Autodesk Inventor part; units mm, degrees
ref_plane "YZ Plane" through (0, 0, 0) normal (1, 0, 0) x (0, 1, 0)
ref_plane "XZ Plane" through (0, 0, 0) normal (0, 1, 0) x (-1, 0, 0)
ref_plane "XY Plane" through (0, 0, 0) normal (0, 0, 1) x (1, 0, 0)
sketch "Sketch1" plane through (0, 0, 0) normal (0, 1, 0) x (-1, 0, 0)
  line L0 (101.6, -101.6) -> (-101.6, -101.6)
  line L1 (-101.6, -101.6) -> (-101.6, 101.6)
  line L2 (-101.6, 101.6) -> (101.6, 101.6)
  line L3 (101.6, 101.6) -> (101.6, -101.6)
  line L4 (96.6, -96.6) -> (-96.6, -96.6)
  line L5 (-96.6, -96.6) -> (-96.6, 96.6)
  line L6 (-96.6, 96.6) -> (96.6, 96.6)
  line L7 (96.6, 96.6) -> (96.6, -96.6)
  line L8 (101.6, 101.6) -> (-40.4, 101.6)
  circle A0 centre (0, 0) radius 86.4
  circle A1 centre (0, 0) radius 109.3376
  line L9 (-40.4, 101.6) -> (-101.6, 40.4)
  line L10 (-45.4, 101.6) -> (-101.6, 45.4)
  line L11 (96.6, 96.6) -> (96.6, 101.6)
  line L12 (-45.4, 101.6) -> (-35.4, 101.6)
  line L13 (-35.4, 101.6) -> (-35.4, 96.6)
  line L14 (-35.4, 96.6) -> (-45.4, 96.6)
  line L15 (-45.4, 96.6) -> (-45.4, 101.6)
  circle A2 centre (0, 0) radius 111.3376
  point P0 (96.6, 51.2168)
  point P1 (101.6, 40.4)
  point P2 (101.6, -40.4)
  point P3 (96.6, -51.2168)
  point P4 (-96.6, 45.4)
  point P5 (-45.4, 96.6)
  dimension "d0" = 203.2
  dimension "d1" = 203.2
  dimension "d2" = 101.6
  dimension "d3" = 101.6
  dimension "d4" = 5
  dimension "d5" = 5
  dimension "d6" = 5
  dimension "d7" = 5
  dimension "d10" = 142
  dimension "d12" = 61.2
  dimension "d14" = 172.8
  dimension "d15" = 5
  dimension "d16" = 5
  dimension "d17" = 10
  dimension "d34" = 2
extrude "Extrusion1" add sketch "Sketch1" along normal blind 3 contours A2 L7 L4 | L4 A1 L7 A2 | L4 A1 L5 L9 L6 L7 | A2 L5 A1 L4 | L4 L5 A2 | A1 L6 A2 L7 | A2 L6 L7
sketch "Sketch5" plane through (0, 3, 0) normal (0, 1, 0) x (1, 0, 0)
  line L0 (-96.6, -96.6) -> (45.4, -96.6)
  circle A0 centre (0, 0) radius 86.4
  line L1 (96.6, -45.4) -> (96.6, 96.6)
  line L2 (96.6, 0) -> (89.1, 0)
  line L3 (89.1, 0) -> (89.1, 10)
  line L4 (89.1, 10) -> (96.6, 10)
  line L5 (96.6, 10) -> (96.6, 0)
  line L6 (89.1, 0) -> (96.6, 0)
  line L7 (96.6, 0) -> (96.6, -10)
  line L8 (96.6, -10) -> (89.1, -10)
  line L9 (89.1, -10) -> (89.1, 0)
  line L10 (0, 0) -> (96.6, 0)
  point P0 (10, -96.6)
  dimension "d52" = 7.5
  dimension "d53" = 7.5
  dimension "d54" = 10
  dimension "d55" = 10
extrude "Extrusion4" add sketch "Sketch5" along normal blind 15 contours L3 L4 L1 L2 | L2 L1 L8 L9
sketch "Sketch7" plane through (89.1, 3, 10) normal (0, 0, 1) x (1, 0, 0)
  line L0 (2, 10) -> (5.5, 10)
  line L1 (5.5, 10) -> (5.5, 3)
  line L2 (5.5, 3) -> (2, 3)
  line L3 (2, 3) -> (2, 10)
  line L4 (7.5, 0) -> (7.5, 15)
  line L5 (0, 0) -> (0, 15)
  line L6 (0, 15) -> (7.5, 15)
  point P0 (-89.1, -3)
  dimension "d56" = 3.5
  dimension "d57" = 2
  dimension "d58" = 2
  dimension "d59" = 5
  dimension "d60" = 7
extrude "Extrusion6" cut sketch "Sketch7" against normal through all
fillet "Fillet7" radius 3.175 2 edges at (96.6, 18, 0) (89.1, 18, 0)
sketch "Sketch8" plane through (0, 3, 0) normal (0, 1, 0) x (1, 0, 0)
  arc A0 (-101.6, -98.425) -> (-98.425, -101.6) centre (-98.425, -98.425) ccw
  line L0 (44.0849, 101.6) -> (-98.425, 101.6)
  line L1 (-101.6, 98.425) -> (-101.6, -98.425)
  line L2 (-101.6, -46.1) -> (-101.6, -76.6)
  line L3 (-96.6, -96.6) -> (-96.6, 96.6)
  line L4 (-96.6, -46.1) -> (-96.6, -76.6)
  line L5 (-101.6, -76.6) -> (-96.6, -76.6)
  line L6 (-101.6, -46.1) -> (-96.6, -46.1)
  line L7 (-98.425, -101.6) -> (101.6, -101.6)
  line L8 (0, 0) -> (-101.6, 0)
  line L9 (-101.6, 46.1) -> (-101.6, 76.6)
  line L10 (-96.6, 46.1) -> (-96.6, 76.6)
  line L11 (-101.6, 76.6) -> (-96.6, 76.6)
  line L12 (-101.6, 46.1) -> (-96.6, 46.1)
  line L13 (-96.6, -76.6) -> (-90.1, -76.6)
  line L14 (-90.1, -76.6) -> (-90.1, -46.1)
  line L15 (-90.1, -46.1) -> (-96.6, -46.1)
  line L16 (-96.6, -46.1) -> (-96.6, -76.6)
  arc A1 (-98.425, 101.6) -> (-101.6, 98.425) centre (-98.425, 98.425) ccw
  line L17 (-101.6, 46.1) -> (-101.6, 76.6)
  line L18 (-96.6, 46.1) -> (-96.6, 76.6)
  line L19 (-101.6, 76.6) -> (-96.6, 76.6)
  line L20 (-101.6, 46.1) -> (-96.6, 46.1)
  line L21 (-96.6, 76.6) -> (-90.1, 76.6)
  line L22 (-90.1, 76.6) -> (-90.1, 46.1)
  line L23 (-90.1, 46.1) -> (-96.6, 46.1)
  line L24 (-96.6, 46.1) -> (-96.6, 76.6)
  line L25 (-96.6, -76.6) -> (-101.6, -76.6)
  line L26 (-101.6, -76.6) -> (-101.6, -74.1)
  line L27 (-101.6, -74.1) -> (-96.6, -74.1)
  line L28 (-96.6, -74.1) -> (-96.6, -76.6)
  line L29 (-96.6, -46.1) -> (-101.6, -46.1)
  line L30 (-101.6, -46.1) -> (-101.6, -48.6)
  line L31 (-101.6, -48.6) -> (-96.6, -48.6)
  line L32 (-96.6, -48.6) -> (-96.6, -46.1)
  line L33 (-96.6, -76.6) -> (-90.1, -76.6)
  line L34 (-90.1, -76.6) -> (-90.1, -74.1)
  line L35 (-90.1, -74.1) -> (-96.6, -74.1)
  line L36 (-96.6, -74.1) -> (-96.6, -76.6)
  line L37 (-96.6, -48.6) -> (-90.1, -48.6)
  line L38 (-90.1, -48.6) -> (-90.1, -46.1)
  line L39 (-90.1, -46.1) -> (-96.6, -46.1)
  line L40 (-96.6, -46.1) -> (-96.6, -48.6)
  line L41 (-96.6, 96.6) -> (-96.6, -96.6)
  line L42 (-90.1, 46.1) -> (-96.6, 46.1)
  line L43 (-96.6, 46.1) -> (-96.6, 48.6)
  line L44 (-96.6, 48.6) -> (-90.1, 48.6)
  line L45 (-90.1, 48.6) -> (-90.1, 46.1)
  line L46 (-90.1, 76.6) -> (-96.6, 76.6)
  line L47 (-96.6, 76.6) -> (-96.6, 74.1)
  line L48 (-96.6, 74.1) -> (-90.1, 74.1)
  line L49 (-90.1, 74.1) -> (-90.1, 76.6)
  point P0 (-98.425, 98.425)
  point P1 (46.1, 101.6)
  point P2 (46.1, 96.6)
  point P3 (76.6, 96.6)
  point P4 (76.6, 101.6)
  point P5 (-46.1, 96.6)
  dimension "d64" = 30.5
  dimension "d65" = 25
  dimension "d66" = 6.5
  dimension "d118" = 2.5
  dimension "d119" = 2.5
  dimension "d120" = 2.5
  dimension "d121" = 2.5
extrude "Extrusion7" cut sketch "Sketch8" against normal through all contours L48 L22 L44 L3 | L37 L14 L35 L3
sketch "Sketch11" plane through (0, 3, 0) normal (0, 1, 0) x (1, 0, 0)
  line L0 (-94, 94) -> (94, 94)
  line L1 (94, 94) -> (94, -94)
  line L2 (94, -94) -> (-94, -94)
  line L3 (-94, -94) -> (-94, 94)
  circle A0 centre (-94, 94) radius 1.5
  circle A1 centre (94, 94) radius 1.5
  circle A2 centre (-94, -94) radius 1.5
  circle A3 centre (94, -39.0849) radius 1.5
  point P0 (0, 0)
  point P1 (0, 0)
  dimension "d98" = 94
  dimension "d99" = 94
  dimension "d100" = 94
  dimension "d101" = 94
  dimension "d102" = 3
  dimension "d103" = 3
  dimension "d104" = 3
  dimension "d105" = 3
extrude "Extrusion8" cut sketch "Sketch11" against normal blind 10 contours L3 A0 L0 | L0 A0 L3 | A1 L1 L0 | L0 L1 A1 | A2 L2 L3 | L3 L2 A2 | A3 L1 | L1 A3
sketch "Sketch12" plane through (0, 3, 0) normal (0, 1, 0) x (1, 0, 0)
  line L0 (-94, 94) -> (94, 94)
  line L1 (94, 94) -> (94, -94)
  line L2 (94, -94) -> (-94, -94)
  line L3 (-94, -94) -> (-94, 94)
  circle A0 centre (-94, 94) radius 2.6
  circle A1 centre (94, 94) radius 2.6
  circle A2 centre (-94, -94) radius 2.6
  circle A3 centre (94, -39.0849) radius 2.6
  point P0 (0, 0)
  point P1 (0, 0)
  point P2 (0, 0)
  dimension "d108" = 94
  dimension "d109" = 94
  dimension "d110" = 94
  dimension "d111" = 94
  dimension "d112" = 5.2
  dimension "d113" = 5.2
  dimension "d114" = 5.2
  dimension "d115" = 5.2
extrude "Extrusion9" cut sketch "Sketch12" against normal blind 1.5 contours L3 A0 L0 | L0 A0 L3 | A1 L1 L0 | L0 L1 A1 | A2 L2 L3 | L3 L2 A2 | A3 L1 | L1 A3
sketch "Sketch13" plane through (0, 3, 0) normal (0, 1, 0) x (1, 0, 0)
  line L0 (94, 96.6) -> (-94, 96.6)
  line L1 (0, 96.6) -> (0, -96.6)
  line L2 (-96.6, -96.6) -> (45.4, -96.6)
  point P0 (0, 0)
ref_plane "Work Plane1" through (0, 3, -96.6) normal (-1, 0, 0) x (0, 0, 1)
sketch "Sketch14" plane through (0, 3, -96.6) normal (-1, 0, 0) x (0, 0, 1)
  line L0 (208.9015, 36.251) -> (-17.5186, 36.251)
  line L1 (-17.5186, 36.251) -> (-17.5186, -18.9911)
  line L2 (-17.5186, -18.9911) -> (208.9015, -18.9911)
  line L3 (208.9015, -18.9911) -> (208.9015, 36.251)
  point P0 (96.6, -3)
extrude "Extrusion10" cut sketch "Sketch14" against normal through all
sketch "Sketch15" plane through (-96.6, 0, -48.6) normal (-1, 0, 0) x (0, 0, 1)
  line L0 (-43.9, 0) -> (-46.9, 0)
  line L1 (141.1, 1.5) -> (141.1, 0)
  line L2 (-43.9, 0) -> (141.1, 0)
  line L3 (141.1, 0) -> (141.1, 1)
  line L4 (141.1, 1) -> (-43.9, 1)
  line L5 (-43.9, 1) -> (-43.9, 0)
  point P0 (48.6, 0)
  dimension "d125" = 1
extrude "Extrusion11" cut sketch "Sketch15" against normal blind 1
equation "\"d1\" = d0"
properties part number "Box_Walls_2"
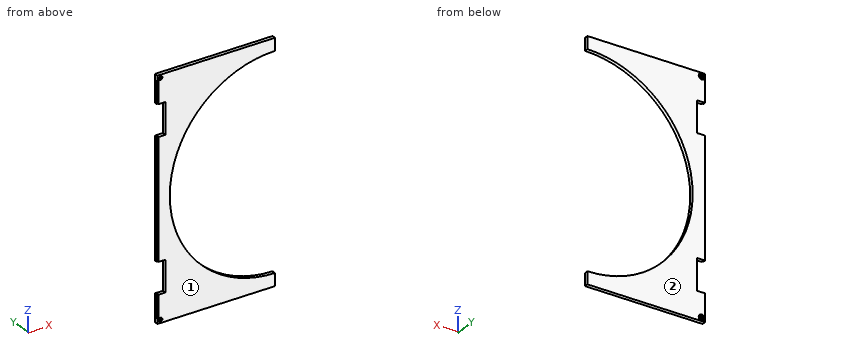
Read the model definition and answer for the solid it produces. Units are mm, in the model's axes. Face numbers are marked on the shaded views. Give positions to 0.01 mm unless a question says otherwise; leave off trailing zeros. Loops run counter-clockwise (first coordinate to the right, second up) from the corner with the lowest first, then second, coordinate; pieces in that order, holes last. Notation, with made-up numbers: (-36.5, -24) - (4.5, -24) arc R28 cw to (4.5, 2) - close; hole circle Ø5 at (46, 25). An arc over 180 degrees is marked (long way). Answer as CSV lines item,"result". Start each with the question number.
1) Find section B-B (x = -57). Write down the section's boundary in (y, z), then the cut area to 3 significant figures.
2) Find section D-D (z = 19.5). Write down the section's boundary in (x, y), then the cut area to 3 significant figures.
3) Straight lines are drawn through the part: L1, parallel to Z at x = -94, y = 1.25; L2, parallel to X at y = 1.05, z = 94; L3, parallel to Z at x = -67, y = 2.3. For each, find the intervals that lie inside material, in ascending order. Write a range as from..to.
4) Each of these flat-tipped pins is pushed along its axis until it touches: pin 1 Ø1.1 at (x, z) = (-96, -86) entering from -Y; pin 2 Ø0.5 at (x, z) = (-96, 79) entering from -Y; pin 3 Ø1.5 at (y, z) = (1.5, 55) entering from -X; pin 4 Ø1.5 at (y, z) = (0.5, -63) entering from +X. Where does it stop, or does it pass through?
5) Determine the mould class of the marked faces 1 and 2 for opening direction Y: released by +Y, released by -Y, zero draft, split by the parting line, or undercut.
6) Find section C-C (z = 0). Write down the section's boundary in (x, y), then the cut area to 3 significant figures.
Findings below:
1,outline,"(0, -96.6) - (3, -96.6) - (3, -64.93) - (0, -64.93) - close; (0, 64.93) - (3, 64.93) - (3, 96.6) - (0, 96.6) - close"
1,area,"190 mm^2"
2,outline,"(-96.6, 1) - (-95.6, 1) - (-95.6, 0) - (-84.17, 0) - (-84.17, 3) - (-96.6, 3) - close"
2,area,"36.3 mm^2"
3,L1,"-96.6..-95.5, -92.5..-74.1, -48.6..48.6, 74.1..92.5, 95.5..96.6"
3,L2,"-96.6..-95.5, -92.5..0"
3,L3,"-96.6..-54.55, 54.55..96.6"
4,pin 1,"y = 0"
4,pin 2,"y = 1"
4,pin 3,"x = -90.1"
4,pin 4,"x = -58.32"
5,face 1,"released by -Y"
5,face 2,"released by +Y"
6,outline,"(-96.6, 1) - (-95.6, 1) - (-95.6, 0) - (-86.4, 0) - (-86.4, 3) - (-96.6, 3) - close"
6,area,"29.6 mm^2"
